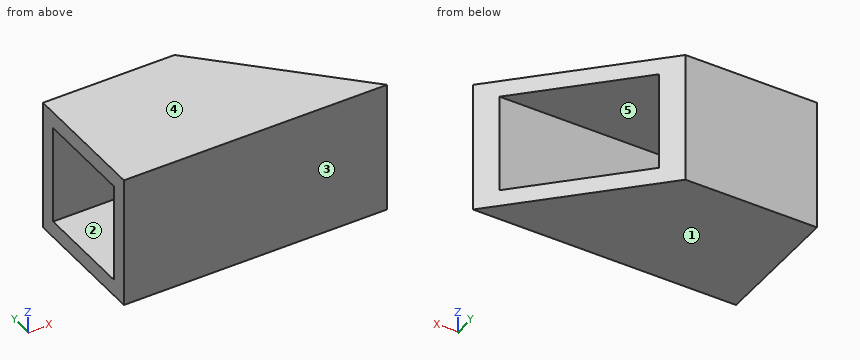
from build123d import *

# Parameters (mm, degrees)
SKETCH1_W           = 25.4
SKETCH1_H           = 25.4
SKETCH1_W_2         = 19.05
SKETCH1_H_2         = 19.05
BOSS_EXTRUDE1_DEPTH = 50.8
CUT_EXTRUDE1_DEPTH  = 26.4


with BuildPart() as part:
    # Sketch1 → Boss-Extrude1 (new body)
    with BuildSketch(Plane(origin=(0, 0, 0), x_dir=(0, 0, -1), z_dir=(1, 0, 0))):
        Rectangle(SKETCH1_W, SKETCH1_H)
        Rectangle(SKETCH1_W_2, SKETCH1_H_2, mode=Mode.SUBTRACT)
    extrude(amount=BOSS_EXTRUDE1_DEPTH)

    # Sketch2 → Cut-Extrude1 (cut, through all)
    with BuildSketch(Plane(origin=(0, 0, -12.7), x_dir=(-1, 0, 0), z_dir=(0, 0, -1))):
        Polygon((-50.8, -12.7), (-25.4, 12.7), (-50.8, 12.7), align=None)
    extrude(amount=-CUT_EXTRUDE1_DEPTH, mode=Mode.SUBTRACT)


solid = part.part
Work out the finished part from the listing and answer in its coordinate system (mm). Face numbers are marked on the shaded views. A direction names the side the tool comes from. Coordinates: 2 decimals unless noted, no trailing zeros. Loops run counter-clockwise (first coordinate to the right, second up) from the corner with the lowest first, then second, coordinate; pieces in that order, holes last. Notation, with made-up numbers: M 5,66 L 43,66 A12 cw 43,81 Z; hole C -35,-30.75 d4. An arc over 180 degrees is marked long. Answer in a Markdown table with one row per item. Add a question column.
1. Find section C-C, the plane z = 0. Write down the section's boundary in (x, y) (3 decimals), then the cut area to 3 significant figures.
2. Find section B-B, the plane x = 21.5. Write down the section's boundary in (y, z) (3 decimals).
3. Find section D-D, the plane x = 37.5. Write down the section's boundary in (y, z) (3 decimals), then the cut area to 3 significant figures.
4. A tool of negligible diameter and unlimited length cuts with its end or side. For the marked faces 4 and 5, from which of +Z, -Z, +X, -X, +Y, -Y can it reach the whole face along a straight path? Write none if from no direction.
5. Flat-ended cylindrical pins translate along their axes: P1, Ø2, axis at y = -9.5, z = -6, coming from the +X side; P2, Ø10, axis at y = 0.5, z = -7, coming from the -X side; P3, Ø8, axis at y = -6, z = -1, coming from the +X side; P4, Ø8, axis at y = 4.5, z = 8, coming from the +X side. Find the tip coordinate at first contact, or state that the pin passes through.
6. Find section A-A, the plane y = -6. Write down the section's boundary in (x, z) (3 decimals), then the cut area to 3 significant figures.
7. The mould has two halves that part along Y. Classify the marked faces 1, 2 and 3: pulls with the +Y half, pulls with the -Y half, needs draft (parallel to the pull), parting line crosses it, or undercut.
8. Consider L1, parallel to Y at x = 9.5, z = -2.25 (3 decimals); L2, parallel to Y at x = 29, z = 9.25 (3 decimals). Determine where each line is inside the solid, lowest interval first.
Reported:
| question | item | result |
|---|---|---|
| 1 | outline | M 0,-12.7 L 50.8,-12.7 L 47.625,-9.525 L 0,-9.525 Z; M 0,9.525 L 28.575,9.525 L 25.4,12.7 L 0,12.7 Z |
| 1 | area | 242 mm^2 |
| 2 | outline | M -12.7,-12.7 L 12.7,-12.7 L 12.7,12.7 L -12.7,12.7 Z; hole M -9.525,-9.525 L 9.525,-9.525 L 9.525,9.525 L -9.525,9.525 Z |
| 3 | outline | M -12.7,-12.7 L 0.6,-12.7 L 0.6,-9.525 L -9.525,-9.525 L -9.525,9.525 L 0.6,9.525 L 0.6,12.7 L -12.7,12.7 Z |
| 3 | area | 145 mm^2 |
| 4 | face 4 | +Z, +X, -X, +Y, -Y |
| 4 | face 5 | +X, -X |
| 5 | P1 | stops at x = 48.6 |
| 5 | P2 | stops at x = 0 |
| 5 | P3 | stops at x = 48.1 |
| 5 | P4 | stops at x = 37.3 |
| 6 | outline | M 0,-12.7 L 44.1,-12.7 L 44.1,-9.525 L 0,-9.525 Z; M 0,9.525 L 44.1,9.525 L 44.1,12.7 L 0,12.7 Z |
| 6 | area | 280 mm^2 |
| 7 | face 1 | needs draft |
| 7 | face 2 | undercut |
| 7 | face 3 | pulls with the -Y half |
| 8 | L1 | y = -12.7 to -9.525, 9.525 to 12.7 |
| 8 | L2 | y = -12.7 to -9.525 |
